Autodesk Inventor part; units mm, degrees
ref_plane "YZ Plane" through (0, 0, 0) normal (1, 0, 0) x (0, 1, 0)
ref_plane "XZ Plane" through (0, 0, 0) normal (0, 1, 0) x (-1, 0, 0)
ref_plane "XY Plane" through (0, 0, 0) normal (0, 0, 1) x (1, 0, 0)
sketch "Sketch1" plane through (0, 0, 0) normal (0, 1, 0) x (-1, 0, 0)
  line L0 (0, 0) -> (0, -32) construction
  line L1 (-3.5, 0) -> (-3.5, -32)
  line L2 (3.5, -32) -> (3.5, 0)
  arc A0 (3.5, 0) -> (-3.5, 0) centre (0, 0) ccw
  arc A1 (-3.5, -32) -> (3.5, -32) centre (0, -32) ccw
  circle A2 centre (0, 0) radius 2.05
  circle A3 centre (0, -32) radius 2.05
  circle A4 centre (0, 0) radius 3.5 construction
  line L3 (-3.5, -4.5) -> (3.5, -4.5)
  line L4 (3.5, -4.5) -> (3.5, -27.5)
  line L5 (3.5, -27.5) -> (-3.5, -27.5)
  line L6 (-3.5, -27.5) -> (-3.5, -4.5)
  line L7 (3.5, -3) -> (-3.5, -3)
  line L8 (3.5, -29) -> (-3.5, -29)
  point P0 (0, -16)
  point P1 (3.5, -16)
  dimension "d0" = 32
  dimension "d1" = 7
  dimension "d2" = 4.1
  dimension "d3" = 4.1
  dimension "d4" = 7
  dimension "d5" = 7
  dimension "d6" = 23
  dimension "d7" = 1.5
  dimension "d8" = 1.5
extrude "Extrusion1" add sketch "Sketch1" along normal blind 14.5
sketch "Sketch3" plane through (0, 14.5, 0) normal (0, 1, 0) x (1, 0, 0)
  line L0 (-3.5, 32) -> (-3.5, 0)
  line L1 (-3.5, 4.5) -> (3.5, 4.5)
  line L2 (3.5, 4.5) -> (3.5, 27.5)
  line L3 (3.5, 27.5) -> (-3.5, 27.5)
  line L4 (-3.5, 27.5) -> (-3.5, 4.5)
  point P0 (0, 0)
  point P1 (-3.5, 16)
  dimension "d15" = 7
  dimension "d16" = 23
extrude "Extrusion2" cut sketch "Sketch3" against normal blind 12.5
sketch "Sketch5" plane through (0, 0, 0) normal (0, -1, 0) x (1, 0, 0)
  line L0 (0, 0) -> (0, -32) construction
  line L1 (-3.5, 0) -> (-3.5, -32)
  line L2 (3.5, -32) -> (3.5, 0)
  arc A0 (3.5, 0) -> (-3.5, 0) centre (0, 0) ccw
  arc A1 (-3.5, -32) -> (3.5, -32) centre (0, -32) ccw
  circle A2 centre (0, 0) radius 2.05
  circle A3 centre (0, -32) radius 2.05
  circle A4 centre (0, 0) radius 3.5 construction
  line L3 (-3.5, -4.5) -> (3.5, -4.5)
  line L4 (3.5, -4.5) -> (3.5, -27.5)
  line L5 (3.5, -27.5) -> (-3.5, -27.5)
  line L6 (-3.5, -27.5) -> (-3.5, -4.5)
  line L7 (3.5, -3) -> (-3.5, -3)
  line L8 (3.5, -29) -> (-3.5, -29)
  point P0 (0, -16)
  point P1 (3.5, -16)
  dimension "d22" = 32
  dimension "d23" = 7
  dimension "d24" = 4.1
  dimension "d25" = 4.1
  dimension "d26" = 7
  dimension "d27" = 7
  dimension "d28" = 23
  dimension "d29" = 1.5
  dimension "d30" = 1.5
extrude "Extrusion3" add sketch "Sketch5" along normal blind 0.9
properties part number "Micro_servo_frame_2"
Input: part model. Units: mm. Frame: model coordinates. A direction names the side the tool comes from. Round coordinates to 2 decimals unless told otherwise and drop trailing zeros. Loops run counter-clockwise (first coordinate to the right, second up) from the corner with the lowest first, then second, coordinate; pieces in that order, holes last. Notation, with made-up numbers: (80.5, -26.5) - (100.5, -26.5) arc R16 cw to (100.5, -12.5) - close; hole circle Ø10 at (30, -13). An arc over 180 degrees is marked (long way). One line per item, written item: value. Start each with the question number.
(1) Ray query, line 1 (Z direction, x = 0, y = -0.7); line 2 (Z direction, x = 1.25, y = 5); line 3 (X direction, y = 9, z = -32). Return the intervals inside material, ascending. Write a range as [from, to].
(2) Section B-B, the plane x = 0. Return loops of the section in (y, z).
(3) Contact query for flat-ended pins moving along their axis: P1, Ø3, axis at x = 2.5, y = 12.5, coming from the -Z side; P2, Ø2, axis at x = 1, z = -17.5, coming from the +Y side; P3, Ø6, axis at y = 9, z = -23.5, coming from the +X side (3 decimals). Output: stop coordinate, or through.
(4) Section A-A, the plane y = 9.5. Return loops of the section in (x, z).
(5) Section C-C, the plane z = -5.5. Return loops of the section in (x, y).
(6) Access query for faces 1 (the flat face through (0, 8, -4.5)), 2 (the flat face through (0, 14.5, -29.7)). Directions: +Z, -Z, +X, -X, +Y, -Y. A direction counts if a zero-diameter tool reaches every point of the face in a straight line with its end or side. Return the directions, or none.
Results below:
1. line 1: [-35.5, -34.05], [-29.95, -2.05], [2.05, 3.5]
1. line 2: [-35.27, -33.62], [-30.38, -27.5], [-4.5, -1.62], [1.62, 3.27]
1. line 3: [-3.5, -2.05], [2.05, 3.5]
2. outline: (-0.9, -35.5) - (14.5, -35.5) - (14.5, -34.05) - (-0.9, -34.05) - close; (-0.9, -29.95) - (14.5, -29.95) - (14.5, -27.5) - (2, -27.5) - (2, -4.5) - (14.5, -4.5) - (14.5, -2.05) - (-0.9, -2.05) - close; (-0.9, 2.05) - (14.5, 2.05) - (14.5, 3.5) - (-0.9, 3.5) - close
3. P1: z = -35.35
3. P2: y = 2
3. P3: through
4. outline: (-3.5, -32) arc R3.5 ccw to (3.5, -32) - (3.5, -27.5) - (-3.5, -27.5) - close; (-3.5, -4.5) - (3.5, -4.5) - (3.5, 0) arc R3.5 ccw to (-3.5, 0) - close; hole circle Ø4.1 at (0, -32); hole circle Ø4.1 at (0, 0)
5. outline: (-3.5, -0.9) - (3.5, -0.9) - (3.5, 2) - (-3.5, 2) - close
6. face 1: +X, -X, +Y
6. face 2: +Z, -Z, +X, -X, +Y
